Here's the drawing with two shaded views (mm, measured from the low corner). I have some questions. A direction names the side the tool comes from. Round coordinates to 2 decimals unless told otherwise and drop trailing zeros. Order: outer loops, then holes, each group sorted by start corner. A loop starts at its lowest first (then second) coordinate and runs counter-clockwise, first axis right, second up. Notation, with made-up numbers: M 22,82 L 55,82 A12 cw 55,100 Z; hole C 37,23 d11. An arc over 180 degrees is marked long. One line per question, with ' | ' between items.
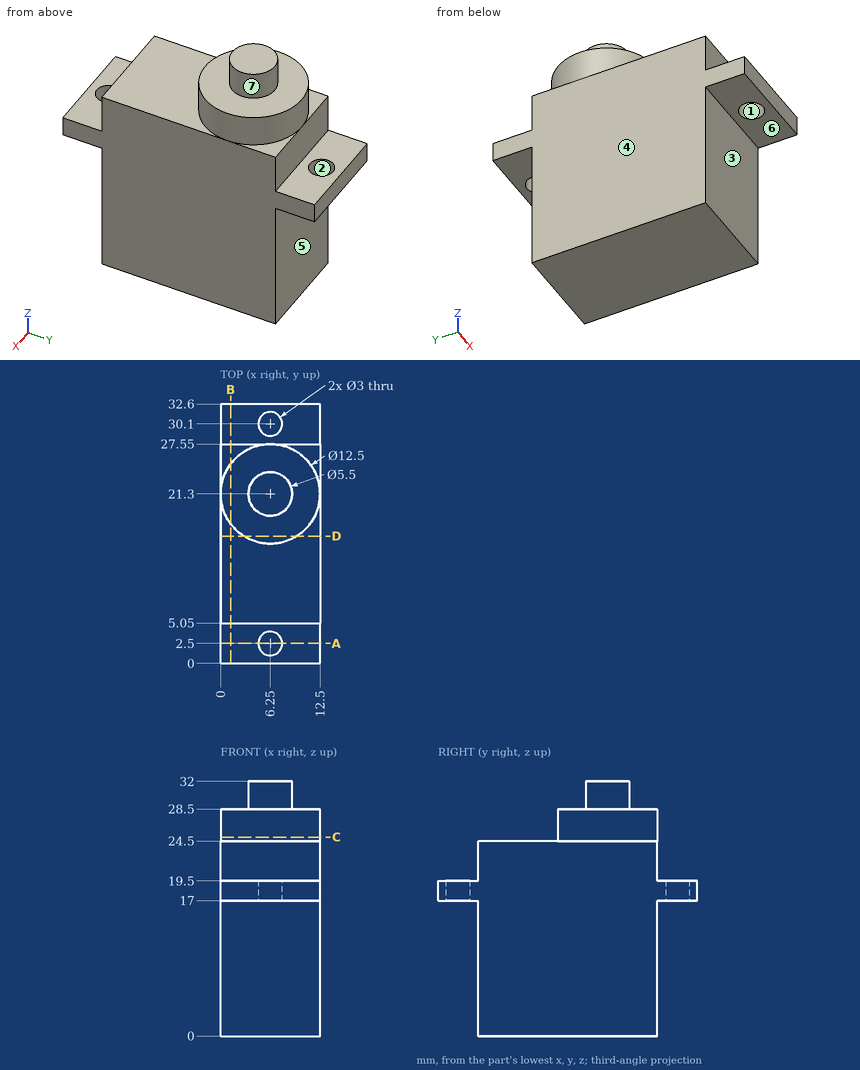
(1) If we section it at D-D on y = 16: Please give me the cut outline in (x, z), plus the area to 3 significant figures.
Final values:
outline: M 0,0 L 12.5,0 L 12.5,24.5 L 9.56,24.5 L 9.56,28.5 L 2.94,28.5 L 2.94,24.5 L 0,24.5 Z | area: 333 mm^2
(2) Thinking about a two-plate mould opening in X: for the marked faces 1, 2, 3 and 4, which applies, released by +X, released by -X, zero draft, split by the parting line, or undercut?
Final values:
face 1: undercut | face 2: undercut | face 3: zero draft | face 4: released by -X
(3) If we section it at C-C on z = 25: Please give me the cut outline in (x, y), plus the area to 3 significant figures.
Final values:
outline: C 6.25,21.3 d12.5 | area: 123 mm^2
(4) If we section it at B-B on x = 1.25: Please give me the cut outline in (y, z), plus the area to 4 significant figures.
Final values:
outline: M 0,17 L 5.05,17 L 5.05,0 L 27.55,0 L 27.55,17 L 32.6,17 L 32.6,19.5 L 27.55,19.5 L 27.55,24.5 L 25.05,24.5 L 25.05,28.5 L 17.55,28.5 L 17.55,24.5 L 5.05,24.5 L 5.05,19.5 L 0,19.5 Z | area: 606.5 mm^2
(5) On a 3-axis mill with a long thin cutter (end or side, diameter ignored), from which of +Z, -Z, +X, -X, +Y, -Y can I reach the whole of each face in a straight line? I mean the marked faces 5, 6 and 7. Say none if no direction works.
Final values:
face 5: -Z, +X, -X, +Y | face 6: -Z, +X, -X, -Y | face 7: +Z
(6) Please list where these lines run through material, in increasing order: probe 1 along Y at (x, z) = (6.25, 19.05); probe 2 along Y at (x, z) = (1.75, 16); probe 3 along Z at (x, y) = (3.75, 5). Write a range as [from, to].
Final values:
probe 1: [0, 1], [4, 28.6], [31.6, 32.6] | probe 2: [5.05, 27.55] | probe 3: [17, 19.5]
(7) Will these pins go through, and if not, where does the flat tip stop? pin 1 Ø4 at (y, z) = (15.5, 23) entering from -X; pin 2 Ø1.5 at (x, y) = (5, 3) entering from -Z; pin 3 Ø4 at (x, z) = (5.5, 9.5) entering from +Y; pin 4 Ø4 at (x, z) = (6, 10.5) entering from -Y.
Final values:
pin 1: x = 0 | pin 2: z = 17 | pin 3: y = 27.55 | pin 4: y = 5.05
(8) If we section it at A-A on y = 2.5: Please give me the cut outline in (x, z), plus the area to 4 significant figures.
Final values:
outline: M 0,17 L 4.75,17 L 4.75,19.5 L 0,19.5 Z; M 7.75,17 L 12.5,17 L 12.5,19.5 L 7.75,19.5 Z | area: 23.75 mm^2
